Here's how the part is built. I have some questions about the finished solid (model axes, mm). Face numbers are marked on the shaded views. A direction names the side the tool comes from. Round coordinates to 2 decimals unless told otherwise and drop trailing zeros. Order: outer loops, then holes, each group sorted by start corner. A loop starts at its lowest first (then second) coordinate and runs counter-clockwise, first axis right, second up. Notation, with made-up numbers: M 17.5,72.25 L 24.5,72.25 A25 ccw 24.5,85.25 Z; hole C 75,-37.5 d2. An arc over 180 degrees is marked long. Write item = value, one per line. Start each with the question number.
Item 1: Please list where these lines run through material, in increasing order: L1, parallel to X at y = 0.5, z = 15.5; L2, parallel to Y at x = -1, z = 49.
Item 2: I want a section at A-A, the plane x = 0. List the corners of the cut face in (y, z) for me, plus the area to 3 significant figures.
Item 3: For the marked faces 1 and 2, which set-ups out of +Z, -Z, +X, -X, +Y, -Y let a thin tool reach every point of the face, with its end or its side?
Item 4: We'd pull the mould along Y, two halves only. Please class the marked faces 3, 4 and 5: pulls with the +Y half, pulls with the -Y half, needs draft (parallel to the pull), parting line crosses it, or undercut.
Item 5: I want a section at B-B, the plane y = -24. List the corners of the cut face in (x, z) for me, plus the area to 3 significant figures.
Item 6: I want a section at C-C, the plane x = 22. List the corners of the cut face in (y, z) for me.
Item 7: I'm going to push flat-ended pins straight in: P1, Ø5, axis at x = 8.5, y = -26.5, coming from the +Z side; P2, Ø14.5, axis at x = 31.5, z = 48.5, coming from the +Y side; P3, Ø5, axis at x = 16, z = 10.5, coming from the +Y side. Where does each tip first touch, or does it pass through?
Item 8: I want a section at D-D, the plane z = 34. List the corners of the cut face in (x, y) for me, plus the area to 3 significant figures.
```python
from build123d import *

# Parameters (mm, degrees)
SKETCH_R             = 29
PAD_DEPTH            = 46
SKETCH001_R          = 35
PAD001_DEPTH         = 2.6
SKETCH002_R          = 33.5
PAD002_DEPTH         = 26.5
SKETCH003_R          = 26.4
POCKET_DEPTH         = 75.101
SKETCH004_R          = 31.3
POCKET001_DEPTH      = 26.75
POCKET002_DEPTH      = 35.001
POCKET002_DEPTH_BACK = -35.001
PAD003_DEPTH         = 10
PAD003_DEPTH_BACK    = 10


with BuildPart() as part:
    # Sketch → Pad (new body)
    with BuildSketch(Plane.XY):
        Circle(SKETCH_R)
    extrude(amount=PAD_DEPTH)

    # Sketch001 (on Face3 of Pad) → Pad001 (join)
    with BuildSketch(Plane.XY.offset(46)):
        Circle(SKETCH001_R)
    extrude(amount=PAD001_DEPTH)

    # Sketch002 (on Face3 of Pad001) → Pad002 (join)
    with BuildSketch(Plane.XY.offset(48.6)):
        Circle(SKETCH002_R)
    extrude(amount=PAD002_DEPTH)

    # Sketch003 (on Face6 of Pad002) → Pocket (cut, through all)
    with BuildSketch(Plane(origin=(0, 0, 0), x_dir=(1, 0, 0), z_dir=(0, 0, -1))):
        Circle(SKETCH003_R)
    extrude(amount=-POCKET_DEPTH, mode=Mode.SUBTRACT)

    # Sketch004 (on Face7 of Pocket) → Pocket001 (cut)
    with BuildSketch(Plane.XY.offset(75.1)):
        Circle(SKETCH004_R)
    extrude(amount=-POCKET001_DEPTH, mode=Mode.SUBTRACT)

    # Sketch005 → Pocket002 (cut, two sides)
    with BuildSketch(Plane.XZ) as pocket002_sk:
        with BuildLine():
            ThreePointArc((-4.55, 71.8), (-6.2, 70.15), (-4.55, 68.5))
            Line((-4.55, 68.5), (4.55, 68.5))
            ThreePointArc((4.55, 68.5), (6.2, 70.15), (4.55, 71.8))
            Line((4.55, 71.8), (-4.55, 71.8))
        make_face()
    extrude(amount=-POCKET002_DEPTH, mode=Mode.SUBTRACT)
    extrude(pocket002_sk.sketch, amount=-POCKET002_DEPTH_BACK, mode=Mode.SUBTRACT)

    # Sketch006 → Pad003 (join, two sides)
    with BuildSketch(Plane.XZ) as pad003_sk:
        with BuildLine():
            Line((26.712868, 17.22326), (29.953513, 17.22326))
            ThreePointArc((29.953513, 17.22326), (34.027862, 18.893168), (35.758251, 22.9422))
            Line((35.758251, 22.9422), (36.710471, 36))
            Line((35.210471, 36), (36.710471, 36))
            Line((35.210471, 41), (35.210471, 36))
            Line((39.035531, 41), (35.210471, 41))
            ThreePointArc((39.035531, 41), (39.500898, 41.188211), (39.704589, 41.647014))
            Line((40.286886, 59.024747), (39.704589, 41.647014))
            ThreePointArc((40.286886, 59.024747), (40.187131, 59.283799), (39.931564, 59.392174))
            Line((37.766381, 59.392174), (39.931564, 59.392174))
            ThreePointArc((37.766381, 59.392174), (37.518605, 59.292543), (37.408773, 59.049117))
            Line((36.783433, 44), (37.408773, 59.049117))
            Line((32.969388, 44), (36.783433, 44))
            ThreePointArc((32.969388, 44), (32.432134, 43.777462), (32.209597, 43.240208))
            Line((32.209597, 43.240208), (32.209597, 22.982091))
            ThreePointArc((29.450765, 20.22326), (31.401553, 21.031303), (32.209597, 22.982091))
            Line((29.450765, 20.22326), (26.712868, 20.22326))
            Line((26.712868, 20.22326), (26.712868, 17.22326))
        make_face()
    extrude(amount=PAD003_DEPTH)
    extrude(pad003_sk.sketch, amount=-PAD003_DEPTH_BACK)


solid = part.part
```
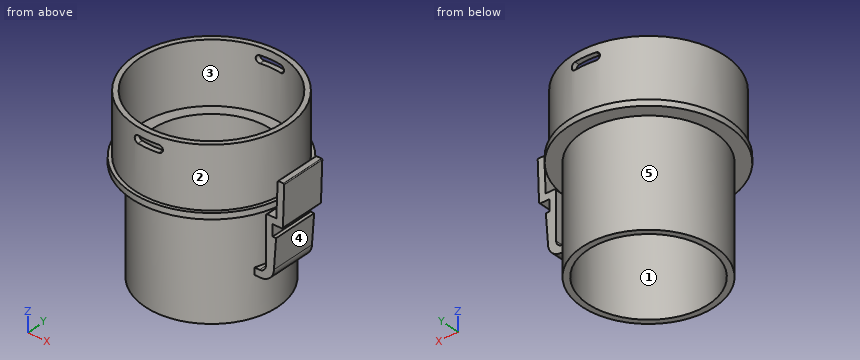
Filled in:
q1.L1 = -29 to -26.4, 26.4 to 29
q1.L2 = -33.49 to -31.28, 31.28 to 33.49
q2.outline = M -35,46 L -29,46 L -29,0 L -26.4,0 L -26.4,48.35 L -31.3,48.35 L -31.3,68.5 L -33.5,68.5 L -33.5,48.6 L -35,48.6 Z; M -33.5,71.8 L -31.3,71.8 L -31.3,75.1 L -33.5,75.1 Z; M 26.4,0 L 29,0 L 29,46 L 35,46 L 35,48.6 L 33.5,48.6 L 33.5,68.5 L 31.3,68.5 L 31.3,48.35 L 26.4,48.35 Z; M 31.3,71.8 L 33.5,71.8 L 33.5,75.1 L 31.3,75.1 Z
q2.area = 384 mm^2
q3.face_1 = +Z, -Z
q3.face_2 = +Z
q4.face_3 = undercut
q4.face_4 = needs draft
q4.face_5 = parting line crosses it
q5.outline = M -25.48,46 L -16.28,46 L -16.28,0 L -11,0 L -11,48.35 L -20.09,48.35 L -20.09,75.1 L -23.37,75.1 L -23.37,48.6 L -25.48,48.6 Z; M 11,0 L 16.28,0 L 16.28,46 L 25.48,46 L 25.48,48.6 L 23.37,48.6 L 23.37,75.1 L 20.09,75.1 L 20.09,48.35 L 11,48.35 Z
q5.area = 730 mm^2
q6.outline = M -27.22,46 L -18.89,46 L -18.89,0 L -14.59,0 L -14.59,48.35 L -22.26,48.35 L -22.26,75.1 L -25.26,75.1 L -25.26,48.6 L -27.22,48.6 Z; M 14.59,0 L 18.89,0 L 18.89,46 L 27.22,46 L 27.22,48.6 L 25.26,48.6 L 25.26,75.1 L 22.26,75.1 L 22.26,48.35 L 14.59,48.35 Z
q7.P1 = 48.35
q7.P2 = 25.24
q7.P3 = 25.67
q8.outline = C 0,0 d58; M 32.21,-10 L 36.56,-10 L 36.56,10 L 32.21,10 Z; hole C 0,0 d52.8
q8.area = 540 mm^2
